Geometry check sheet. Reference: the model listing, model coordinates, mm. Face numbers are marked on the shaded views. A direction names the side the tool comes from. Coordinates: 2 decimals unless noted, no trailing zeros. Loops run counter-clockwise (first coordinate to the right, second up) from the corner with the lowest first, then second, coordinate; pieces in that order, holes last.
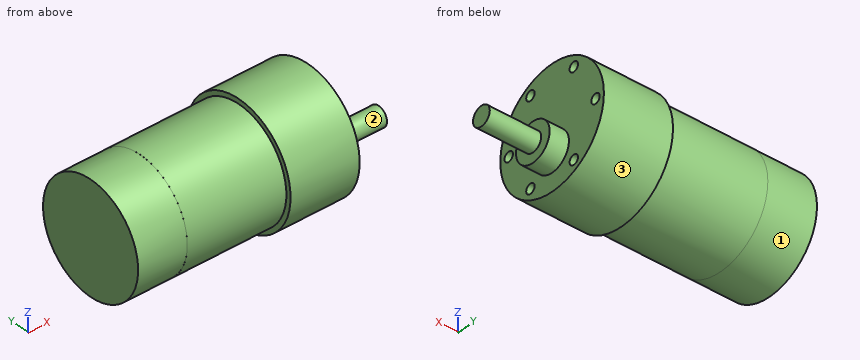
Autodesk Fusion 360 part; units mm, degrees
sketch "Esquisse1" plane through (0, 0, 0) normal (0, 0, 1) x (1, 0, 0) in component "Motor"
  line L0 (0, 0) -> (0, 16.99)
  line L1 (0, 16.99) -> (15.3, 16.99)
  line L2 (15.3, 16.99) -> (15.3, 0)
  line L3 (46.1, 17) -> (46.1, 0)
  line L4 (46.1, 0) -> (67.6, 0) construction
  line L5 (67.6, 0) -> (67.6, 18.5)
  line L6 (67.6, 18.5) -> (46.1, 18.5)
  line L7 (46.1, 18.5) -> (46.1, 17)
  line L8 (0, 0) -> (67.6, 0)
  line L9 (15.3, 16.99) -> (15.3, 17)
  line L10 (15.3, 17) -> (46.1, 17)
  dimension "d2" = 16.99
  dimension "d7" = 15.3
  dimension "d8" = 30.8
  dimension "d10" = 21.5
  dimension "d11" = 18.5
  dimension "d12" = 21.5
  dimension "d13" = 0.01
revolve "Révolution1" add sketch "Esquisse1" angle 360 about axis through (0, 0, 0) along (1, 0, 0) makes body 1 in component "Motor"
sketch "Esquisse2" plane through (67.6, 0, 0) normal (1, 0, 0) x (0, 1, 0) in component "Motor"
  circle A0 centre (0, 0) radius 18.5
  line L0 (0, 0) -> (18.5, 0) construction
  line L1 (0, 0) -> (-15.5, 0) construction
  circle A1 centre (-15.5, 0) radius 1.5
  circle A2 centre (0, 0) radius 15.5 construction
  line L2 (-15.5, 0) -> (-7.75, -13.4234) construction
  circle A3 centre (-7.75, -13.4234) radius 1.5
  circle A4 centre (-7.75, 13.4234) radius 1.5
  line L3 (0, 0) -> (0, -18.5) construction
  circle A5 centre (7.75, 13.4234) radius 1.5
  circle A6 centre (15.5, 0) radius 1.5
  circle A7 centre (7.75, -13.4234) radius 1.5
  line L4 (0, 0) -> (0, -7) construction
  circle A8 centre (0, -7) radius 6
  circle A9 centre (0, -7) radius 3
  dimension "d14" = 15.5
  dimension "d15" = 3
  dimension "d16" = 15.5
  dimension "d17" = 3
  dimension "d18" = 7
  dimension "d19" = 12
  dimension "d20" = 6
  dimension "d27" = 3
  dimension "d28" = 3
  dimension "d29" = 3
  dimension "d30" = 3
extrude "Extrusion3" cut sketch "Esquisse2" against normal blind 10 contours A1 | A3 | A4 | A5 | A6 | A7 bodies 1 in component "Motor"
extrude "Extrusion1" add sketch "Esquisse2" along normal blind 6 contours A8 bodies 1 in component "Motor"
extrude "Extrusion2" add 1 faces at (67.6, -1.8565, -7.7286) along direction (1, 0, 0) blind 22 on bodies 1 bodies 1 in component "Motor"
copy_body "CutPasteBodies1" bodies 1 removing the originals makes body 2 in component "Motor"
component "Motor" placed x (1, 0, 0) y (0, 1, 0) z (0, 0, 1) at (0, 0, 0)
equation "d2 = ( ( 34 / 2 ) * 1 ) * 1 mm - 0.01 mm"
equation "d11 = ( 37 / 2 ) * 1 mm"
equation "d14 = ( 31 / 2 ) * 1 mm"
equation "d17 = d15"
1) Section check C-C on x = 66. Record the cut outline in (y, z), and give its area (3 significant figures).
Data:
outline: circle Ø37 at (0, 0); hole circle Ø3 at (-15.5, 0); hole circle Ø3 at (-7.75, -13.42); hole circle Ø3 at (-7.75, 13.42); hole circle Ø3 at (7.75, -13.42); hole circle Ø3 at (7.75, 13.42); hole circle Ø3 at (15.5, 0)
area: 1,030 mm2
2) Depth check by flat-ended pin: pin 1 (4 mm diameter, centred on x = 64, z = -10.5, fed in from +Y); pin 2 (5 mm diameter, centred on y = -15.5, z = 0, fed in from +X); pin 3 (12 mm diameter, centred on x = 23.5, z = -9, fed in from +Y); pin 4 (10 mm diameter, centred on y = -4.5, z = -3.5, fed in from -X). Enter the tip coordinate at first touch or a pass-through.
Data:
pin 1: stops at y = 16.43
pin 2: stops at x = 67.6
pin 3: stops at y = 16.73
pin 4: stops at x = 0
3) Material ranges on probe 1 along Z at (x, y) = (64.75, -7.75); probe 2 along X at (y, z) = (10.5, 11.5); probe 3 along Z at (x, y) = (60, 7), recorded low to high.
Data:
probe 1: z = -16.8 to -14.92, -11.92 to 11.92, 14.92 to 16.8
probe 2: x = 0 to 67.6
probe 3: z = -17.12 to -14.72, -12.12 to 12.12, 14.72 to 17.12
4) Section check D-D on x = 47. Record the cut outline in (y, z).
Data:
outline: circle Ø37 at (0, 0)
5) Access from +Z, -Z, +X, -X, +Y, -Y to the whole of each face (thin tool, end or side, straight path). Record for the marked faces 1, 2 and 3.
Data:
face 1: -X
face 2: +X
face 3: +X, -X
